Here's how the part is built. I have some questions about the finished solid (model axes, mm). A direction names the side the tool comes from. Give positions to 0.01 mm unless a question says otherwise; leave off trailing zeros. Write each loop counter-clockwise with the first axis right and the second up, starting at its lowest first coordinate (ties: lowest second). Pieces come first, ordered by that corner, then holes. Notation, with made-up numbers: (-19.5, -36.75) - (24.5, -36.75) arc R23 cw to (24.5, -13.75) - close; hole circle Ø1 at (35.25, 14). An arc over 180 degrees is marked (long way). Write each question's results on one line, items separated by ' | '. Start each with the question number.
Item 1: Which directions (+Z, -Z, +X, -X, +Y, -Y) give clear straight access to the entire face, cutting with the end or side of a thin tool? Please do faces 1 (the flat face through (17.9, -8.5, -1.3)), 2 (the flat face through (17.9, -8.6, 1.3)), 3 (the flat face through (18.5, -8.3, -2.1)).
Item 2: Please list where these lines run through material, in increasing order: line 1 along Y through (x, z) = (18.75, 0); line 2 along Y through (x, z) = (17.9, 0); line 3 along Z through (x, y) = (19.3, -0.75).
Item 3: Suppose I cut it at A-A on x = 18.95. List the corners of the cut face in (y, z) for me.
Item 4: Suppose I cut it at B-B on z = 0. List the corners of the cut face in (x, y) for me, then the cut area to 3 significant figures.
Item 5: We'd pull the mould along Z, two halves only. Please class faces 4 (the flat face through (19, -9.35, 5)), 5 (the conical face through (17.435, 7.978, 0.334)), 6 (the flat face through (19, -5, 9.35)), 7 (the flat face through (18, -9.05, 0)): +Z half, -Z half, draft (parallel to the pull), parting line (faces both ways), or undercut.
Item 6: Will this pin go through, and if not, where does the flat tip stop? P1, Ø1.1, axis at x = 18.5, z = 0, coming from the -Y side.
```python
from build123d import *

# Parameters (mm, degrees)
SKETCH_1_R      = 3
EXTRUDE_1_DEPTH = 1.2
CHAMFER_1_SIZE  = 0.5
EXTRUDE_START   = 1
SKETCH_2_R      = 3
EXTRUDE_2_DEPTH = 1


with BuildPart() as part:
    # Эскиз1 → Бобышка-Вытянуть1 (new body)
    with BuildSketch(Plane(origin=(18.5, 0, 0), x_dir=(0, 0, -1), z_dir=(1, 0, 0))):
        with BuildLine():
            Line((1.3, -9.05), (-1.3, -9.05))
            Line((-1.3, -9.05), (-1.3, -8.417392708))
            Line((-1.3, -8.417392708), (-1.3, -8.248181618))
            ThreePointArc((-1.3, -8.248181618), (0, 8.35), (1.3, -8.248181618))
            Line((1.3, -8.248181618), (1.3, -8.417392708))
            Line((1.3, -8.417392708), (1.3, -9.05))
        make_face()
        Circle(SKETCH_1_R, mode=Mode.SUBTRACT)
    extrude(amount=-EXTRUDE_1_DEPTH)

    # Фаска1
    chamfer_1_edges = [part.edges().sort_by_distance(p)[0] for p in [
        (17.3, 8.35, 0),
    ]]
    chamfer(chamfer_1_edges, length=CHAMFER_1_SIZE)

    # Эскиз2 → Бобышка-Вытянуть2 (add)
    with BuildSketch(Plane(origin=(18.5, 0, 0), x_dir=(0, 0, -1), z_dir=(1, 0, 0)).offset(EXTRUDE_START)):
        with BuildLine():
            Line((1.5, -9.05), (-1.5, -9.05))
            Line((-1.5, -9.05), (-1.5, -9.35))
            Line((-1.5, -9.35), (-9.35, -9.35))
            Line((-9.35, -9.35), (-9.35, 0))
            ThreePointArc((-9.35, 0), (0, 9.35), (9.35, 0))
            Line((9.35, 0), (9.35, -9.35))
            Line((9.35, -9.35), (1.5, -9.35))
            Line((1.5, -9.35), (1.5, -9.05))
        make_face()
        Circle(SKETCH_2_R, mode=Mode.SUBTRACT)
    extrude(amount=-EXTRUDE_2_DEPTH)


solid = part.part
```
Checked values:
1) face 1: -Z, -X, -Y | face 2: +Z, -X, -Y | face 3: -X
2) line 1: y = -9.05 to -3, 3 to 9.35 | line 2: y = -9.05 to -3, 3 to 8.35 | line 3: z = -9.35 to -2.9, 2.9 to 9.35
3) outline: (-9.35, -9.35) - (0, -9.35) arc R9.35 ccw to (0, 9.35) - (-9.35, 9.35) - (-9.35, 1.5) - (-9.05, 1.5) - (-9.05, -1.5) - (-9.35, -1.5) - close; hole circle Ø6 at (0, 0)
4) outline: (17.3, -9.05) - (19.5, -9.05) - (19.5, -3) - (17.3, -3) - close; (17.3, 3) - (19.5, 3) - (19.5, 9.35) - (18.5, 9.35) - (18.5, 8.35) - (17.8, 8.35) - (17.3, 7.85) - close | area: 26.0 mm^2
5) face 4: draft | face 5: parting line | face 6: +Z half | face 7: undercut
6) P1: stops at y = -9.05
